Check sheet for the modelled part. Datum: model origin and axes. Units: mm. Give positions to 0.01 mm unless a question says otherwise; leave off trailing zeros. Order: outer loops, then holes, each group sorted by start corner. A loop starts at its lowest first (then second) coordinate and runs counter-clockwise, first axis right, second up. Notation, with made-up numbers: (19.5, 63) -> (36.5, 63) arc R31 cw to (36.5, 99) -> close; hole circle Ø6 at (-40, 44.5). An arc over 180 degrees is marked (long way). One line per question, with ' | ' between items.
```python
from build123d import *

# Parameters (mm, degrees)
F0_W     = 137.5
F0_H     = 195
F0_W_2   = 60
F0_H_2   = 10
F1_DEPTH = 15
F2_W     = 137.5
F2_H     = 15
F3_DEPTH = 7.5
F4_R     = 2.5
F5_DEPTH = 7.5
F6_R     = 3


with BuildPart() as f1:
    # F0 (on Front) → F1 (new body)
    with BuildSketch(Plane.XZ):
        with Locations((-1.555176, 3.066924)):
            Rectangle(F0_W, F0_H)
        with Locations((-34.030074, -82.667378)):
            Rectangle(F0_W_2, F0_H_2, mode=Mode.SUBTRACT)
        with Locations((-34.030074, -68.667378)):
            Rectangle(F0_W_2, F0_H_2, mode=Mode.SUBTRACT)
        with Locations((-34.030074, -54.667378)):
            Rectangle(F0_W_2, F0_H_2, mode=Mode.SUBTRACT)
        with Locations((-34.030074, -40.667378)):
            Rectangle(F0_W_2, F0_H_2, mode=Mode.SUBTRACT)
        with Locations((-34.030074, -26.667378)):
            Rectangle(F0_W_2, F0_H_2, mode=Mode.SUBTRACT)
        with Locations((-34.030074, -12.667378)):
            Rectangle(F0_W_2, F0_H_2, mode=Mode.SUBTRACT)
        with Locations((-34.030074, 1.332622)):
            Rectangle(F0_W_2, F0_H_2, mode=Mode.SUBTRACT)
        with Locations((31.969926, -82.667378)):
            Rectangle(F0_W_2, F0_H_2, mode=Mode.SUBTRACT)
        with Locations((31.969926, -68.667378)):
            Rectangle(F0_W_2, F0_H_2, mode=Mode.SUBTRACT)
        with Locations((31.969926, -54.667378)):
            Rectangle(F0_W_2, F0_H_2, mode=Mode.SUBTRACT)
        with Locations((31.969926, -40.667378)):
            Rectangle(F0_W_2, F0_H_2, mode=Mode.SUBTRACT)
        with Locations((31.969926, -26.667378)):
            Rectangle(F0_W_2, F0_H_2, mode=Mode.SUBTRACT)
        with Locations((31.969926, -12.667378)):
            Rectangle(F0_W_2, F0_H_2, mode=Mode.SUBTRACT)
        with Locations((31.969926, 1.332622)):
            Rectangle(F0_W_2, F0_H_2, mode=Mode.SUBTRACT)
        with Locations((-34.030074, 15.332622)):
            Rectangle(F0_W_2, F0_H_2, mode=Mode.SUBTRACT)
        with Locations((-34.030074, 29.332622)):
            Rectangle(F0_W_2, F0_H_2, mode=Mode.SUBTRACT)
        with Locations((-34.030074, 43.332622)):
            Rectangle(F0_W_2, F0_H_2, mode=Mode.SUBTRACT)
        with Locations((-34.030074, 57.332622)):
            Rectangle(F0_W_2, F0_H_2, mode=Mode.SUBTRACT)
        with Locations((-34.030074, 71.332622)):
            Rectangle(F0_W_2, F0_H_2, mode=Mode.SUBTRACT)
        with Locations((31.969926, 15.332622)):
            Rectangle(F0_W_2, F0_H_2, mode=Mode.SUBTRACT)
        with Locations((31.969926, 29.332622)):
            Rectangle(F0_W_2, F0_H_2, mode=Mode.SUBTRACT)
        with Locations((31.969926, 43.332622)):
            Rectangle(F0_W_2, F0_H_2, mode=Mode.SUBTRACT)
        with Locations((31.969926, 57.332622)):
            Rectangle(F0_W_2, F0_H_2, mode=Mode.SUBTRACT)
        with Locations((31.969926, 71.332622)):
            Rectangle(F0_W_2, F0_H_2, mode=Mode.SUBTRACT)
    extrude(amount=F1_DEPTH)

    # F2 (on Front) → F3 (cut)
    with BuildSketch(Plane.XZ):
        with Locations((-1.555176, 93.066924)):
            Rectangle(F2_W, F2_H)
    extrude(amount=F3_DEPTH, mode=Mode.SUBTRACT)

    # F4 (on face) → F5 (cut, through all)
    with BuildSketch(Plane.XZ.offset(15)):
        with Locations((24.194824, 91.566924)):
            Circle(F4_R)
    extrude(amount=-F5_DEPTH, mode=Mode.SUBTRACT)

    # F6
    f6_edges = [f1.edges().sort_by_distance(p)[0] for p in [
        (-1.555176, -15, 100.566924),
        (-70.305176, -15, 3.066924),
        (67.194824, -15, 3.066924),
        (-1.555176, -15, -94.433076),
    ]]
    fillet(f6_edges, radius=F6_R)


solid = f1.part
```
Q1. Section check A-A (z = -25.5). Enter the section's corners in (x, y), and give its area (3 significant figures).
Result sheet:
outline: (-70.31, -12) arc R3 ccw to (-67.31, -15) -> (-64.03, -15) -> (-64.03, 0) -> (-70.31, 0) -> close; (-4.03, -15) -> (1.97, -15) -> (1.97, 0) -> (-4.03, 0) -> close; (61.97, -15) -> (64.19, -15) arc R3 ccw to (67.19, -12) -> (67.19, 0) -> (61.97, 0) -> close | area: 259 mm2
Q2. Thickness scan on line 1 (X direction, y = -6.25, z = 18.5); line 2 (X direction, y = -13, z = 16.5); line 3 (Z direction, x = 1.5, y = -5.25). Record the ranges inside material, lowest first.
Result sheet:
line 1: x = -70.31 to -64.03, -4.03 to 1.97, 61.97 to 67.19 | line 2: x = -70.13 to -64.03, -4.03 to 1.97, 61.97 to 67.02 | line 3: z = -94.43 to 85.57
Q3. Depth check by flat-ended pin: pin 1 Ø3 at (x, z) = (-23, 45.5) entering from -Y; pin 2 Ø1 at (x, y) = (-17, -5) entering from +Z. Enter the tip coordinate at first touch or a pass-through.
Result sheet:
pin 1: passes through | pin 2: stops at z = 85.57
Q4. Mould release check, pull along X, two halves, no side actions. Record for faces 1 (the face through (32, -7, -73.667)), 2 (the face through (-70.305, -6, 2)), 3 (the face through (-3, -10, 100.567)): pulls with the +X half, pulls with the -X half, needs draft (parallel to the pull), parting line crosses it, or undercut.
Result sheet:
face 1: undercut | face 2: pulls with the -X half | face 3: needs draft
Q5. Section check B-B (x = 29). Count the separate pieces of the cut face and the enclosed holes in it, and give its area (3 significant figures).
Result sheet:
separate pieces: 13 | enclosed holes: 0 | area: 1,010 mm2
